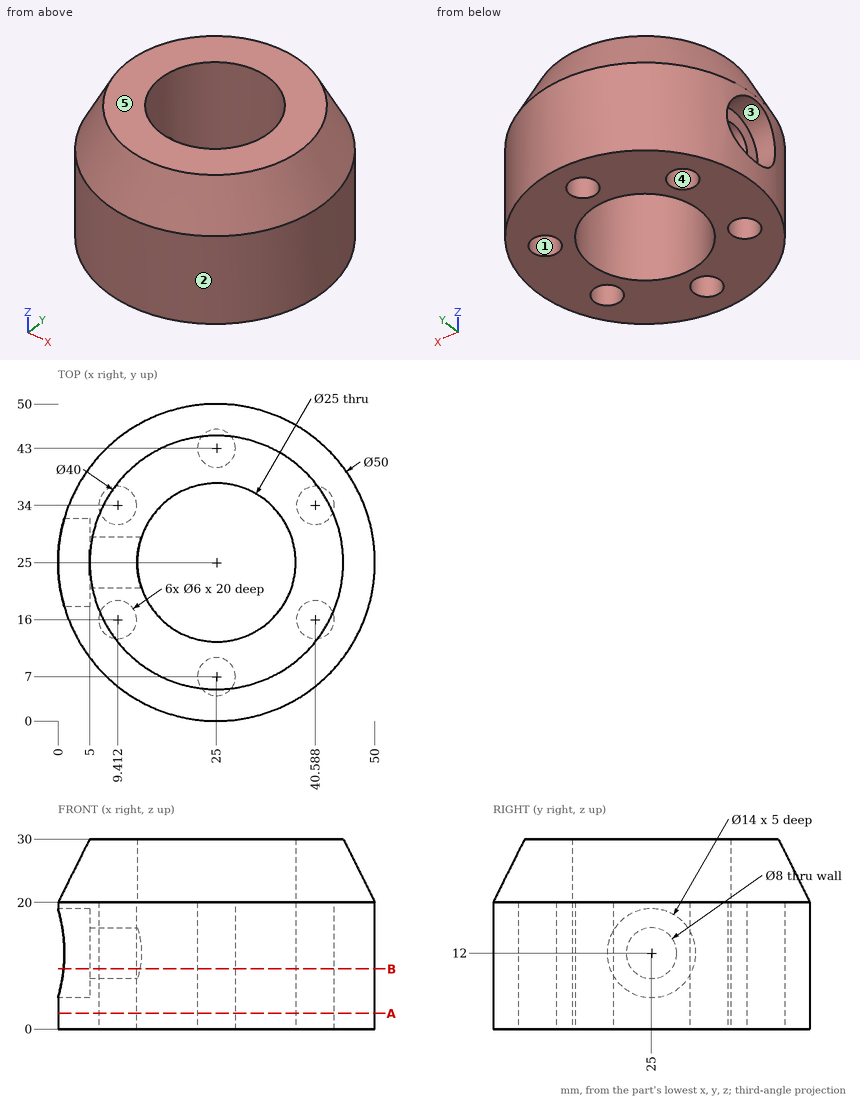
The figure shows three views and two pictorial views of one solid part (mm, origin at its lowest corner). Answer the questions. A direction names the side the tool comes from. Give positions to 0.01 mm unless a question says otherwise; leave off trailing zeros. Loops run counter-clockwise (first coordinate to the right, second up) from the corner with the lowest first, then second, coordinate; pieces in that order, holes last. Notation, with made-up numbers: (-15.5, 82.5) -> (31.5, 82.5) arc R27 ccw to (31.5, 105.5) -> close; hole circle Ø4 at (33, 8). An arc over 180 degrees is marked (long way). Use a Markdown table: item, result. Add a question column.
1. Determine the mould class of the marked faces 3, 4 and 5 for opening direction Z: released by +Z, released by -Z, zero draft, split by the parting line, or undercut.
2. Flat-ended cylindrical pins translate along their axes: pin 1 Ø12 at (y, z) = (35.5, 15.5) entering from +X; pin 2 Ø22.5 at (x, y) = (25, 25) entering from +Z; pin 3 Ø9.5 at (x, y) = (25, 43) entering from -Z; pin 4 Ø3 at (x, y) = (24, 7) entering from -Z. Find the tip coordinate at first contact, or state that the pin passes through.
3. Section A-A on z = 2.5 is taken. Determine the outline of the cut face in (x, y).
4. For the marked faces 1 and 2, determine the directions among +Z, -Z, +X, -X, +Y, -Y from which every point of the face is accessible in a straight line to the end or side of a thin tool.
5. Find the intervals of material crossed by probe 1 along Y at (x, z) = (25, 13); probe 2 along X at (y, z) = (33, 6) (1 decimal); probe 3 along Y at (x, z) = (27, 22.5) (1 decimal), in increasing order.
6. Section B-B on z = 9.5 is taken. Determine the outline of the cut face in (x, y).
Results below:
| question | item | result |
|---|---|---|
| 1 | face 3 | undercut |
| 1 | face 4 | zero draft |
| 1 | face 5 | released by +Z |
| 2 | pin 1 | stops at x = 49.59 |
| 2 | pin 2 | passes through |
| 2 | pin 3 | stops at z = 0 |
| 2 | pin 4 | stops at z = 20 |
| 3 | outline | circle Ø50 at (25, 25); hole circle Ø6 at (9.41, 16); hole circle Ø6 at (9.41, 34); hole circle Ø25 at (25, 25); hole circle Ø6 at (25, 7); hole circle Ø6 at (25, 43); hole circle Ø6 at (40.59, 16); hole circle Ø6 at (40.59, 34) |
| 4 | face 1 | -Z |
| 4 | face 2 | +Z, -Z |
| 5 | probe 1 | y = 0 to 4, 10 to 12.5, 37.5 to 40, 46 to 50 |
| 5 | probe 2 | x = 1.3 to 6.6, 12.2 to 15.4, 34.6 to 37.8, 43.4 to 48.7 |
| 5 | probe 3 | y = 1.3 to 12.7, 37.3 to 48.7 |
| 6 | outline | (0.87, 18.46) arc R25 ccw (long way) to (0.87, 31.54) -> (5, 31.54) -> (5, 28.12) -> (12.9, 28.12) arc R12.5 cw (long way) to (12.9, 21.88) -> (5, 21.88) -> (5, 18.46) -> close; hole circle Ø6 at (9.41, 16); hole circle Ø6 at (9.41, 34); hole circle Ø6 at (25, 7); hole circle Ø6 at (25, 43); hole circle Ø6 at (40.59, 16); hole circle Ø6 at (40.59, 34) |
